Design review of the part built by this model. Coordinates are the model's own, in mm. Coordinates: 2 decimals unless noted, no trailing zeros. Loops run counter-clockwise (first coordinate to the right, second up) from the corner with the lowest first, then second, coordinate; pieces in that order, holes last. Notation, with made-up numbers: (37, -34) - (89, -34) arc R25 ccw to (89, -21) - close; hole circle Ø1 at (83, -33). An arc over 180 degrees is marked (long way). One line per question, with ' | ' between items.
from build123d import *

# Parameters (mm, degrees)
SKETCH1_W           = 150
SKETCH1_H           = 21.4
BOSS_EXTRUDE2_DEPTH = 2
SKETCH2_W           = 5
SKETCH2_H           = 2
BOSS_EXTRUDE3_DEPTH = 2.5
LPATTERN1_COUNT     = 15
LPATTERN1_PITCH     = 10
SKETCH3_W           = 5
SKETCH3_H           = 2
BOSS_EXTRUDE4_DEPTH = 2.5
LPATTERN2_COUNT     = 15
LPATTERN2_PITCH     = 10


with BuildPart() as part:
    # Sketch1 → Boss-Extrude2 (new body)
    with BuildSketch(Plane.XY):
        with Locations((75, 10.7)):
            Rectangle(SKETCH1_W, SKETCH1_H)
    extrude(amount=BOSS_EXTRUDE2_DEPTH)

    # Sketch2 → Boss-Extrude3 (add)
    with BuildSketch(Plane(origin=(0, 21.4, 0), x_dir=(1, 0, 0), z_dir=(0, 1, 0))):
        with Locations((7.5, -1)):
            Rectangle(SKETCH2_W, SKETCH2_H)
    boss_extrude3 = extrude(amount=BOSS_EXTRUDE3_DEPTH)

    # LPattern1: Boss-Extrude3 ×15
    with Locations(*[(i * LPATTERN1_PITCH, 0, 0) for i in range(1, LPATTERN1_COUNT)]):
        add(boss_extrude3)

    # Sketch3 → Boss-Extrude4 (add)
    with BuildSketch(Plane(origin=(0, 0, 0), x_dir=(-1, 0, 0), z_dir=(0, -1, 0))):
        with Locations((-7.5, -1)):
            Rectangle(SKETCH3_W, SKETCH3_H)
    boss_extrude4 = extrude(amount=BOSS_EXTRUDE4_DEPTH)

    # LPattern2: Boss-Extrude4 ×15
    with Locations(*[(i * LPATTERN2_PITCH, 0, 0) for i in range(1, LPATTERN2_COUNT)]):
        add(boss_extrude4)


solid = part.part
Q1. Take a section at A-A (x = 12). Give the boundary of the cut face in (y, z).
Returned:
outline: (0, 0) - (21.4, 0) - (21.4, 2) - (0, 2) - close
Q2. To check wall thickness, follow line 1 along Y through (x, z) = (72, 1.35). State the ranges of the line that lie inside material, in increasing order.
Returned:
line 1: y = 0 to 21.4
Q3. For pin 1 (5 mm diameter, centred on x = 18, y = 6.5, fed in from -Z); pin 2 (1 mm diameter, centred on x = 143, z = 1, fed in from -Y); pin 3 (1 mm diameter, centred on y = -1, z = 1.5, fed in from -X), all flat-tipped, find the tip position at first contact; note any pin that passes through.
Returned:
pin 1: stops at z = 0 | pin 2: stops at y = 0 | pin 3: stops at x = 5
